```python
from build123d import *

# Parameters (mm, degrees)
BOSS_EXTRUDE1_DEPTH = 3
SKETCH5_W           = 43
SKETCH5_H           = 24
CUT_EXTRUDE4_DEPTH  = 3
FILLET1_R           = 10


with BuildPart() as part:
    # Sketch1 → Boss-Extrude1 (new body)
    with BuildSketch(Plane(origin=(0, 0, 0), x_dir=(1, 0, 0), z_dir=(0, 1, 0))):
        Polygon((12.75, -17), (12.75, 17), (12.75, 21.75), (2.75, 21.75), (2.75, 17), (-40.25, 17), (-40.25, 21.75), (-50.25, 21.75), (-50.25, 17), (-50.25, -17), (-50.25, -21.75), (-40.25, -21.75), (-40.25, -17), (2.75, -17), (2.75, -21.75), (12.75, -21.75), align=None)
    extrude(amount=BOSS_EXTRUDE1_DEPTH)

    # Sketch5 → Cut-Extrude4 (cut)
    with BuildSketch(Plane(origin=(0, 3, 0), x_dir=(1, 0, 0), z_dir=(0, 1, 0))):
        with Locations((-18.75, 0)):
            Rectangle(SKETCH5_W, SKETCH5_H)
    extrude(amount=-CUT_EXTRUDE4_DEPTH, mode=Mode.SUBTRACT)

    # Fillet1
    fillet1_edges = [part.edges().sort_by_distance(p)[0] for p in [
        (2.75, 1.5, 12),
        (-40.25, 1.5, 12),
        (-40.25, 1.5, -12),
        (2.75, 1.5, -12),
    ]]
    fillet(fillet1_edges, radius=FILLET1_R)


solid = part.part
```
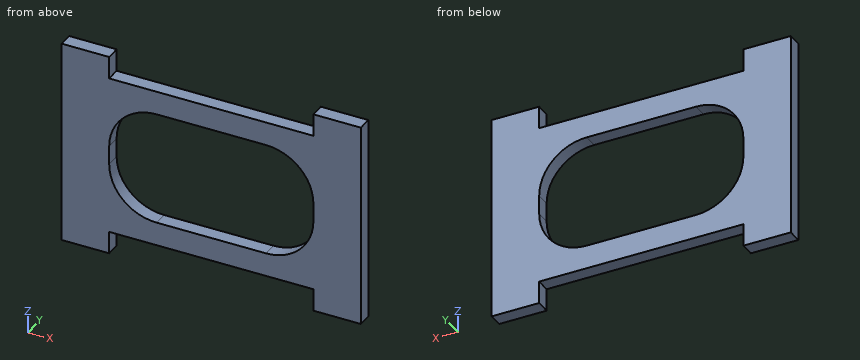
Here's how the part is built. I have some questions about the finished solid (model axes, mm). Coordinates: 2 decimals unless noted, no trailing zeros. Order: outer loops, then holes, each group sorted by start corner. A loop starts at its lowest first (then second) coordinate and runs counter-clockwise, first axis right, second up. Notation, with made-up numbers: (20.25, 82) - (70.25, 82) arc R22 cw to (70.25, 89) - close; hole circle Ø4 at (65, 30). An arc over 180 degrees is marked (long way). One line per question, with ' | ' between items. Start each with the question number.
1. If we section it at B-B (y = 0.7): Write out the boundary of the cut face in (x, z).
2. I'm going to push flat-ended pins straight in: pin 1 Ø0.9 at (x, y) = (-20.5, 1) entering from +Z; pin 2 Ø1.5 at (x, y) = (-17.5, 1) entering from -Z. Where does each tip first touch, or does it pass through?
3. If we section it at A-A (x = -28): Write out the boundary of the cut face in (y, z), and give its area (3 significant figures).
4. Please list where these lines run through material, in increasing order: line 1 along Z through (x, y) = (-10, 2.25); line 2 along X through (y, z) = (0.4, -20); line 3 along Z through (x, y) = (0, 2.55). Write a range as [from, to].
5. If we section it at C-C (z = -9): Write out the boundary of the cut face in (x, y), and give its area (3 significant figures).
Model answer:
1) outline: (-50.25, -21.75) - (-40.25, -21.75) - (-40.25, -17) - (2.75, -17) - (2.75, -21.75) - (12.75, -21.75) - (12.75, 21.75) - (2.75, 21.75) - (2.75, 17) - (-40.25, 17) - (-40.25, 21.75) - (-50.25, 21.75) - close; hole (-40.25, -2) arc R10 ccw to (-30.25, -12) - (-7.25, -12) arc R10 ccw to (2.75, -2) - (2.75, 2) arc R10 ccw to (-7.25, 12) - (-30.25, 12) arc R10 ccw to (-40.25, 2) - close
2) pin 1: stops at z = 17 | pin 2: stops at z = -17
3) outline: (0, -17) - (3, -17) - (3, -12) - (0, -12) - close; (0, 12) - (3, 12) - (3, 17) - (0, 17) - close | area: 30.0 mm²
4) line 1: z = [-17, -12], [12, 17] | line 2: x = [-50.25, -40.25], [2.75, 12.75] | line 3: z = [-17, -8.89], [8.89, 17]
5) outline: (-50.25, 0) - (-37.39, 0) - (-37.39, 3) - (-50.25, 3) - close; (-0.11, 0) - (12.75, 0) - (12.75, 3) - (-0.11, 3) - close | area: 77.2 mm²
